Part model, mm, in its own coordinate system. A direction names the side the tool comes from. Coordinates: 2 decimals unless noted, no trailing zeros. Loops run counter-clockwise (first coordinate to the right, second up) from the corner with the lowest first, then second, coordinate; pieces in that order, holes last. Notation, with made-up numbers: (20.5, 44.25) - (25.5, 44.25) arc R23 cw to (25.5, 54.25) - close; hole circle Ø6 at (-0.75, 52.25). An arc over 180 degrees is marked (long way). Use a Markdown table: item, result. Add a question column.
1) Band-saw the part on B-B (z = 2.5). Give the cut face in (x, y).
2) Band-saw the part on C-C (z = 4.1). Give the cut face in (x, y).
3) Band-saw the part on A-A (x = 0). Give the cut face in (y, z).
4) Probe probe 1 along X at (y, z) = (-2.9, 2.5); probe 2 along Z at (x, y) = (0, -2.85); probe 3 along Y at (x, z) = (3.75, 0.55). List the from-to ranges inside material, lowest first. Write a range as [from, to].
5) Band-saw the part on D-D (x = -3). Give the cut face in (y, z).
6) Tool access for faces 1 (the face through (0, -2.75, 2)), 2 (the face through (0, 2, 2)): list every direction of +Z, -Z, +X, -X, +Y, -Y with a clear straight run to the whole face (end or side of a thin tool).
from build123d import *

# Parameters (mm, degrees)
SKETCH1_W           = 8
SKETCH1_H           = 4
BOSS_EXTRUDE1_DEPTH = 5
SKETCH2_R           = 2
BOSS_EXTRUDE2_DEPTH = 1
SKETCH5_R           = 1
CUT_EXTRUDE1_DEPTH  = 0.25


with BuildPart() as part:
    # Sketch1 → Boss-Extrude1 (new body)
    with BuildSketch(Plane.XY):
        Rectangle(SKETCH1_W, SKETCH1_H)
    extrude(amount=BOSS_EXTRUDE1_DEPTH)

    # Sketch2 → Boss-Extrude2 (add)
    with BuildSketch(Plane(origin=(0, -2, 0), x_dir=(-1, 0, 0), z_dir=(0, -1, 0))):
        with Locations((0, -2.5)):
            Circle(SKETCH2_R)
    extrude(amount=BOSS_EXTRUDE2_DEPTH)

    # Sketch5 → Cut-Extrude1 (cut)
    with BuildSketch(Plane(origin=(0, -3, 0), x_dir=(-1, 0, 0), z_dir=(0, -1, 0))):
        with Locations((0, -2.5)):
            Circle(SKETCH5_R)
    extrude(amount=-CUT_EXTRUDE1_DEPTH, mode=Mode.SUBTRACT)


solid = part.part
Answer block:
| question | item | result |
|---|---|---|
| 1 | outline | (-4, -2) - (-2, -2) - (-2, -3) - (-1, -3) - (-1, -2.75) - (1, -2.75) - (1, -3) - (2, -3) - (2, -2) - (4, -2) - (4, 2) - (-4, 2) - close |
| 2 | outline | (-4, -2) - (-1.2, -2) - (-1.2, -3) - (1.2, -3) - (1.2, -2) - (4, -2) - (4, 2) - (-4, 2) - close |
| 3 | outline | (-3, 0.5) - (-2, 0.5) - (-2, 0) - (2, 0) - (2, 5) - (-2, 5) - (-2, 4.5) - (-3, 4.5) - (-3, 3.5) - (-2.75, 3.5) - (-2.75, 1.5) - (-3, 1.5) - close |
| 4 | probe 1 | [-2, -1], [1, 2] |
| 4 | probe 2 | [0.5, 1.5], [3.5, 4.5] |
| 4 | probe 3 | [-2, 2] |
| 5 | outline | (-2, 0) - (2, 0) - (2, 5) - (-2, 5) - close |
| 6 | face 1 | -Y |
| 6 | face 2 | +Z, -Z, +X, -X, +Y |
